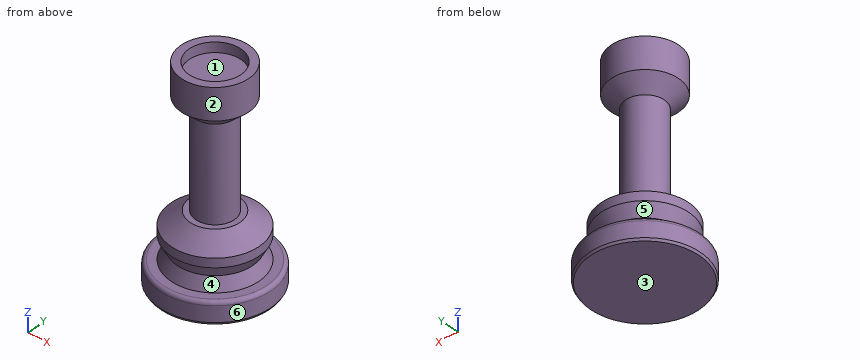
```python
from build123d import *


with BuildPart() as f1:
    # F0 (on Front) → F1 (revolve)
    with BuildSketch(Plane.XZ):
        with BuildLine():
            Line((0, 0), (15.367, 0))
            Line((15.367, 0), (15.748, 0.635))
            Line((15.748, 0.635), (15.748, 5.08))
            ThreePointArc((15.748, 5.08), (15.45042, 5.79842), (14.732, 6.096))
            Line((14.732, 6.096), (12.446, 6.096))
            Line((12.446, 6.096), (10.668, 9.398))
            Line((10.668, 9.398), (12.446, 12.7))
            Line((12.446, 12.7), (12.446, 15.24))
            Line((12.446, 15.24), (7.029734, 19.05))
            Line((7.029734, 19.05), (5.461, 19.05))
            Line((5.461, 19.05), (5.461, 45.528467))
            Line((5.461, 45.528467), (9.538582, 49.266249))
            Line((9.538582, 49.266249), (9.538582, 58.08828))
            Line((9.538582, 58.08828), (7.322641, 58.08828))
            Line((7.322641, 58.08828), (7.322641, 55.292979))
            Line((7.322641, 55.292979), (0, 55.292979))
            Line((0, 55.292979), (0, 0))
        make_face()
    revolve(axis=Axis((0, 0, 27.646489), (0, 0, -1)))


solid = f1.part
```
The listing builds one solid part. Answer for the finished solid, in the listing's coordinates (mm). Face numbers are marked on the shaded views. A direction names the side the tool comes from. Round coordinates to 2 decimals unless told otherwise and drop trailing zeros. Order: outer loops, then holes, each group sorted by start corner. A loop starts at its lowest first (then second) coordinate and runs counter-clockwise, first axis right, second up. Notation, with made-up numbers: (18, 88.25) -> (31, 88.25) arc R17 ccw to (31, 110.25) -> close; hole circle Ø11 at (81, 78). An arc over 180 degrees is marked (long way). Answer as CSV lines item,"result".
Q1. Which of the six approach directions +Z, -Z, +X, -X, +Y, -Y give full straight-line access (tool end or side, diameter ignored) to the marked faces 5 and 6?
Computed values:
face 5,"none"
face 6,"+Z, -Z"
Q2. A cutting plane is placed at D-D on z = 51. Determine the outline of the cut face in (x, y), plus the area to 3 significant figures.
Computed values:
outline,"circle Ø19.08 at (0, 0)"
area,"286 mm^2"
Q3. For a pull along Z with two mould halves and no side action, classify the marked faces 1, 2, 3 and 4 as +Z half, -Z half, draft (parallel to the pull), parting line (faces both ways), or undercut.
Computed values:
face 1,"+Z half"
face 2,"draft"
face 3,"-Z half"
face 4,"undercut"
Q4. A cutting plane is placed at A-A on z = 30. Determine the outline of the cut face in (x, y).
Computed values:
outline,"circle Ø10.92 at (0, 0)"
Q5. Consider line 1 (X direction, y = 0, z = 56); line 2 (Z direction, x = -11.5, y = -1). Determine where each line is inside the solid, lowest interval first. Write a range as from..to.
Computed values:
line 1,"x = -9.54..-7.32, 7.32..9.54"
line 2,"z = 0..7.77, 11.02..15.87"
Q6. Given pin 1 (8 mm diameter, centred on x = -12, z = 7, fed in from -Y); pin 2 (7.5 mm diameter, centred on x = 0, y = 0.5, fed in from +Z); pin 3 (12 mm diameter, centred on y = -2, z = 26, fed in from +X); pin 4 (1 mm diameter, centred on x = 6, z = 42.5, fed in from -Y), each flat-ended and moving along its own axis, determine where each tip first touches the part or whether it passes through.
Computed values:
pin 1,"stops at y = -13.31"
pin 2,"stops at z = 55.29"
pin 3,"stops at x = 5.46"
pin 4,"passes through"
